from build123d import *

# Parameters (mm, degrees)
F0_W      = 1016
F0_H      = 635
F1_DEPTH  = 12.7
F2_W      = 190.9023970366
F2_H      = 72.670340538
F2_W_2    = 110.4675829411
F2_H_2    = 338.8325423002
F2_W_3    = 187.6850500703
F2_H_3    = 73.4205134213
F3_DEPTH  = 25.4
F4_W      = 260.4392468929
F4_H      = 36.7102567106
F4_H_2    = 39.9852208793
F4_W_2    = 25.2980589867
F4_H_3    = 0.1311842352
F5_DEPTH  = 25.4
F6_W      = 29.0026068687
F6_H      = 39.524897933
F6_W_2    = 26.9005596638
F6_H_2    = 22.802144289
F6_W_3    = 26.5395641327
F6_H_3    = 40.0708019733
F6_W_4    = 25.1247286797
F6_H_4    = 17.9900527
F7_DEPTH  = 12.7
F8_W      = 8.947044611
F8_H      = 11.3622983918
F8_W_2    = 8.928835392
F8_H_2    = 11.6621851921
F8_W_3    = 8.7315738201
F8_H_3    = 12.1389040723
F9_DEPTH  = 2.54
F10_R     = 4.1746501932
F10_R_2   = 4.2690475455
F11_DEPTH = 0.762
F12_R     = 0.76199
F13_W     = 21.8863785267
F13_H     = 167.8882390261
F14_DEPTH = 15.24


# Not quite as in the source:
# - a fillet or chamfer is up to 0.001 mm smaller than in the source, because OpenCascade refuses the exact size


with BuildPart() as f1:
    # F0 (on Top) → F1 (new body)
    with BuildSketch(Plane.XY):
        Rectangle(F0_W, F0_H)
    extrude(amount=-F1_DEPTH)

    # F2 (on face) → F3 (join)
    with BuildSketch(Plane.XY):
        Polygon((-73.4143704176, 178.6967664957), (-73.4143704176, 106.0264259577), (-73.4143704176, 41.7220070958), (-2.6750040706, 41.7220070958), (-2.6750040706, 178.8768768311), (-73.4143704176, 178.8768768311), align=None)
        with Locations((-168.8655689359, 142.3615962267)):
            Rectangle(F2_W, F2_H)
        with Locations((-385.0155323744, 9.5723941922)):
            Rectangle(F2_W_2, F2_H_2)
        with Locations((-166.5967218578, -121.2908085436)):
            Rectangle(F2_W_3, F2_H_3)
        Polygon((-72.7541968226, -84.5805518329), (-72.7541968226, -158.0010652542), (0, -158.0010652542), (0, -20.846195519), (-72.7541968226, -20.846195519), align=None)
    extrude(amount=F3_DEPTH)

    # F4 (on face) → F5 (join)
    with BuildSketch(Plane.XY.offset(25.4)):
        with Locations((-130.2196234465, -139.6459368989)):
            Rectangle(F4_W, F4_H)
        with Locations((-133.8504105806, 157.6813366264)):
            Rectangle(F4_W, F4_H_2)
        Polygon((-362.4670803547, 0.1311842352), (-362.4670803547, 0), (-387.7651393414, 0), (-387.7651393414, -49.7534926981), (-362.2698187828, -49.7534926981), (-362.2698187828, 0.1311842352), align=None)
        with Locations((-375.116109848, 0.0655921176)):
            Rectangle(F4_W_2, F4_H_3)
        Polygon((-387.9624009132, 0), (-387.7651393414, 0), (-387.7651393414, 0.1311842352), (-362.4670803547, 0.1311842352), (-362.4670803547, 49.8846769333), (-387.9624009132, 49.8846769333), align=None)
    extrude(amount=F5_DEPTH)

    # F6 (on face) → F7 (join)
    with BuildSketch(Plane.XY.offset(25.4)):
        Polygon((-343.3714807034, -149.6838778257), (-343.3714807034, -125.3397166729), (-400.9214937687, -125.3397166729), (-429.9241006374, -125.3397166729), (-429.9241006374, -149.6838778257), align=None)
        with Locations((-415.4227972031, -105.5772677064)):
            Rectangle(F6_W, F6_H)
        with Locations((-360.9930127859, -97.2158908844)):
            Rectangle(F6_W_2, F6_H_2)
        Polygon((-342.8669273853, 141.4012908936), (-342.8669273853, 169.8563098907), (-429.579526186, 169.8563098907), (-429.579526186, 141.4012908936), (-403.0399620533, 141.4012908936), align=None)
        with Locations((-416.3097441196, 121.3658899069)):
            Rectangle(F6_W_3, F6_H_3)
        with Locations((-367.4284219742, 110.3255152702)):
            Rectangle(F6_W_4, F6_H_4)
    extrude(amount=F7_DEPTH)

    # F8 (on face) → F9 (join)
    with BuildSketch(Plane.XY.offset(50.8)):
        with Locations((-383.2916170359, -1.178430859)):
            Rectangle(F8_W, F8_H)
        with Locations((-383.4979832172, 15.6762860715)):
            Rectangle(F8_W_2, F8_H_2)
        with Locations((-383.3993524313, -16.8637591414)):
            Rectangle(F8_W_3, F8_H_3)
    extrude(amount=F9_DEPTH)

    # F10 (on face) → F11 (join)
    with BuildSketch(Plane.XY.offset(53.34)):
        with Locations((-383.3409547806, -17.0078240335)):
            Circle(F10_R)
        with Locations((-383.3993524313, 15.7660990953)):
            Circle(F10_R_2)
    extrude(amount=F11_DEPTH)

    # F12 (radius 0.762 in the source; OpenCascade refuses exactly that, so slightly less here)
    f12_edges = [f1.edges().sort_by_distance(p)[0] for p in [
        (-387.515605, -17.007824, 54.102),
        (-387.6684, 15.766099, 54.102),
    ]]
    fillet(f12_edges, radius=F12_R)

    # F13 (on face) → F14 (join)
    with BuildSketch(Plane.XY):
        with Locations((-318.8385516405, 11.3731846213)):
            Rectangle(F13_W, F13_H)
    extrude(amount=F14_DEPTH)


solid = f1.part
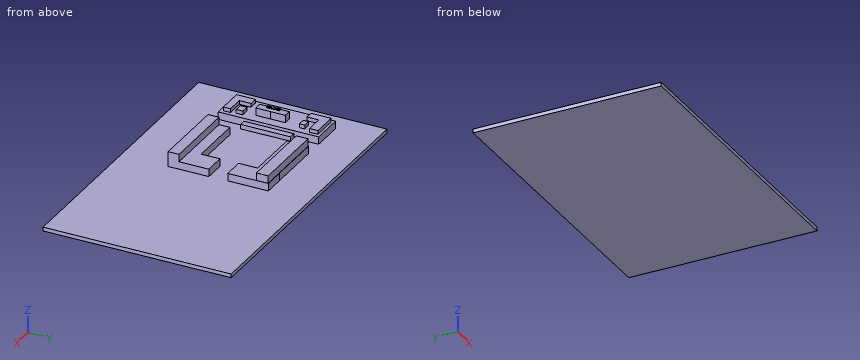
Source: CAD feature listing. Evaluate the final solid. Frame: model axes, mm. Round coordinates to 2 decimals unless told otherwise and drop trailing zeros. Loops run counter-clockwise (first coordinate to the right, second up) from the corner with the lowest first, then second, coordinate; pieces in that order, holes last. Notation, with made-up numbers: (-7, 75.5) - (32, 75.5) arc R26 cw to (32, 89.5) - close; hole circle Ø6 at (21.5, 37.5). An arc over 180 degrees is marked (long way). Write item = value, one per line. Start each with the question number.
Item 1: Section query C-C on x = 125. Output: boundary loops of the cut face in (y, z), plus the area to 3 significant figures.
Item 2: Section query A-A on x = -209.5. Output: boundary loops of the cut face in (y, z).
Item 3: Material intervals for line 1 (X direction, y = -96, z = 5.5); line 2 (Y direction, x = -15, z = 9.5); line 3 (X direction, y = -24.5, z = 3), sorted ascending.
Item 4: Section query B-B on y = 225. Output: boundary loops of the cut face in (x, z), plus the area to 3 significant figures.
Item 5: First-contact query: pin 1 Ø8.5 at (y, z) = (29.5, 40.5) entering from -X; pin 2 Ø15 at (x, z) = (-105.5, 20) entering from -Y; pin 3 Ø10 at (x, z) = (-376.5, 34) entering from -Y. Flat tips, straight axial feed; report the tip coordinate or a pass-through.
Results list:
q1.outline = (-317.5, -12.7) - (317.5, -12.7) - (317.5, 0) - (-317.5, 0) - close
q1.area = 8,060 mm²
q2.outline = (-317.5, -12.7) - (317.5, -12.7) - (317.5, 0) - (178.7, 0) - (178.7, 25.4) - (177.67, 25.4) - (177.67, 50.8) - (137.69, 50.8) - (137.69, 25.4) - (106.03, 25.4) - (106.03, 0) - (-84.58, 0) - (-84.58, 25.4) - (-121.29, 25.4) - (-121.29, 50.8) - (-158, 50.8) - (-158, 0) - (-317.5, 0) - close
q3.line_1 = -440.25 to -329.78, -260.44 to 0
q3.line_2 = -158 to -20.85, 41.72 to 178.88
q3.line_3 = -440.25 to -307.9, -72.75 to 0
q4.outline = (-508, -12.7) - (508, -12.7) - (508, 0) - (-508, 0) - close
q4.area = 12,900 mm²
q5.pin_1 = -387.96
q5.pin_2 = -158
q5.pin_3 = -149.68
